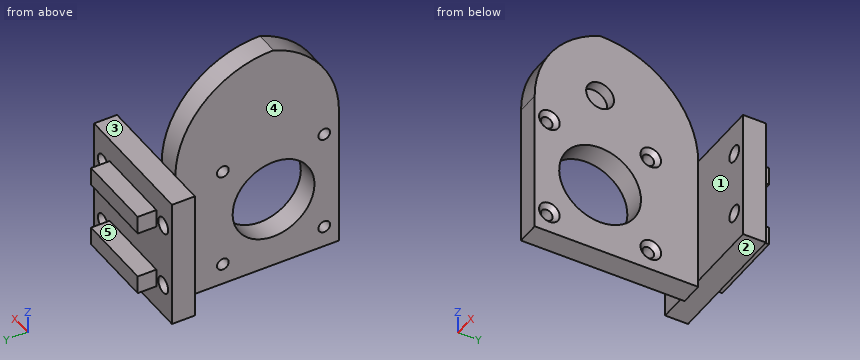
from build123d import *

# Parameters (mm, degrees)
CROQUIS1_W                                           = 40
CROQUIS1_H                                           = 40
SALIENTE_EXTRUIR1_DEPTH                              = 7
CROQUIS3_W                                           = 5.6
CROQUIS3_H                                           = 5.7
SALIENTE_EXTRUIR3_DEPTH                              = 40
CROQUIS19_W                                          = 8
CROQUIS19_H                                          = 40
CORTAR_EXTRUIR5_DEPTH                                = 5.7
CROQUIS20_R                                          = 2.5
CORTAR_EXTRUIR6_DEPTH                                = 7
CROQUIS21_W                                          = 7
CROQUIS21_H                                          = 72
SALIENTE_EXTRUIR4_DEPTH                              = 50
CROQUIS22_R                                          = 12.5
CORTAR_EXTRUIR7_DEPTH                                = 7
AVELLANADO_PARA_TORNILLO_CON_CABEZA_PLAN_D           = 3.6
AVELLANADO_PARA_TORNILLO_CON_CABEZA_PLAN_CSINK_D     = 6.3
AVELLANADO_PARA_TORNILLO_CON_CABEZA_PLAN_CSINK_ANGLE = 90
CROQUIS25_R                                          = 4.25
CORTAR_EXTRUIR8_DEPTH                                = 3.5
REDONDEO1_R                                          = 30
REDONDEO2_R                                          = 30


# Some blends are built 0.0001 mm under size
with BuildPart() as part:
    # Croquis1 → Saliente-Extruir1 (new body)
    with BuildSketch(Plane(origin=(0, 0, 0), x_dir=(1, 0, 0), z_dir=(0, 1, 0))):
        Rectangle(CROQUIS1_W, CROQUIS1_H)
    extrude(amount=SALIENTE_EXTRUIR1_DEPTH)

    # Croquis3 → Saliente-Extruir3 (add)
    with BuildSketch(Plane.ZY.offset(20)):
        with Locations((10, 9.85)):
            Rectangle(CROQUIS3_W, CROQUIS3_H)
        with Locations((-10, 9.85)):
            Rectangle(CROQUIS3_W, CROQUIS3_H)
    extrude(amount=-SALIENTE_EXTRUIR3_DEPTH)

    # Croquis19 → Cortar-Extruir5 (cut)
    with BuildSketch(Plane(origin=(0, 12.7, 0), x_dir=(1, 0, 0), z_dir=(0, 1, 0))):
        with Locations((-16, 0)):
            Rectangle(CROQUIS19_W, CROQUIS19_H)
        with Locations((16, 0)):
            Rectangle(CROQUIS19_W, CROQUIS19_H)
    extrude(amount=-CORTAR_EXTRUIR5_DEPTH, mode=Mode.SUBTRACT)

    # Croquis20 → Cortar-Extruir6 (cut)
    with BuildSketch(Plane(origin=(0, 7, 0), x_dir=(1, 0, 0), z_dir=(0, 1, 0))):
        with Locations(Location((-15.5, 10, 0), (0, 0, 270))):
            Circle(CROQUIS20_R)
        with Locations(Location((15.5, 10, 0), (0, 0, 270))):
            Circle(CROQUIS20_R)
        with Locations(Location((15.5, -10, 0), (0, 0, 270))):
            Circle(CROQUIS20_R)
        with Locations(Location((-15.5, -10, 0), (0, 0, 270))):
            Circle(CROQUIS20_R)
    extrude(amount=-CORTAR_EXTRUIR6_DEPTH, mode=Mode.SUBTRACT)

    # Croquis21 → Saliente-Extruir4 (add)
    with BuildSketch(Plane.XZ):
        with Locations((-6.5, 14)):
            Rectangle(CROQUIS21_W, CROQUIS21_H)
    extrude(amount=SALIENTE_EXTRUIR4_DEPTH)

    # Croquis22 → Cortar-Extruir7 (cut)
    with BuildSketch(Plane(origin=(-3, 0, 0), x_dir=(0, 0, -1), z_dir=(1, 0, 0))):
        with Locations((0, -30)):
            Circle(CROQUIS22_R)
    extrude(amount=-CORTAR_EXTRUIR7_DEPTH, mode=Mode.SUBTRACT)

    # Avellanado para tornillo con cabeza plana de M31 (through all)
    with Locations(Plane(origin=(-3, -14.5, 15.5), x_dir=(0, 0, 1), z_dir=(1, 0, 0))):
        with Locations((0, 0), (-31, 0), (-31, 31), (0, 31)):
            CounterSinkHole(AVELLANADO_PARA_TORNILLO_CON_CABEZA_PLAN_D / 2, AVELLANADO_PARA_TORNILLO_CON_CABEZA_PLAN_CSINK_D / 2, counter_sink_angle=AVELLANADO_PARA_TORNILLO_CON_CABEZA_PLAN_CSINK_ANGLE)

    # Croquis25 → Cortar-Extruir8 (cut)
    with BuildSketch(Plane(origin=(-3, 0, 0), x_dir=(0, 0, -1), z_dir=(1, 0, 0))):
        with Locations((-30, -30)):
            Circle(CROQUIS25_R)
    extrude(amount=-CORTAR_EXTRUIR8_DEPTH, mode=Mode.SUBTRACT)

    # Redondeo1
    redondeo1_edges = [part.edges().sort_by_distance(p)[0] for p in [
        (-6.5, 0, 50),
    ]]
    fillet(redondeo1_edges, radius=REDONDEO1_R - 0.0001)  # a hair under: the kernel refuses the full size

    # Redondeo2
    # the kernel refuses this fillet: 30 mm, written as the material it takes off along each edge
    with BuildSketch(Plane(origin=(67.710766507, -50, 50), x_dir=(0, 1, 0), z_dir=(-1, 0, 0))) as redondeo2_piece_1:
        with BuildLine():
            CenterArc((30, 28.284306603), REDONDEO2_R, 180, 70.528981937)
            Line((0, 28.284306603), (-0.6, 28.284306603))
            Line((-0.6, 28.284306603), (-0.6, 0))
            Line((-0.6, 0), (0, -0.6))
            ThreePointArc((0, -0.6), (10.00005, -0.6), (19.800102, -0.565686132))
            Line((19.800102, -0.565686132), (20.0001, 0))
        make_face()
    extrude(amount=148.421533013, mode=Mode.SUBTRACT)


solid = part.part
Here's how the part is built. I have some questions about the finished solid (model axes, mm). Face numbers are marked on the shaded views. A direction names the side the tool comes from. Coordinates: 2 decimals unless noted, no trailing zeros. Write each loop counter-clockwise with the first axis right and the second up, starting at its lowest first coordinate (ties: lowest second). Pieces come first, ordered by that corner, then holes. Notation, with made-up numbers: (-4, 49.25) - (2, 49.25) arc R17 cw to (2, 57.25) - close; hole circle Ø1 at (26, -31). An arc over 180 degrees is marked (long way). Use one line per item in the form item = value.
1) Suppose I cut it at D-D, the plane y = -14.5. Write out the boundary of the cut face in (x, z), plus the area to 3 significant figures.
Solved:
outline = (-10, -22) - (-3, -22) - (-3, -18.65) - (-4.35, -17.3) - (-10, -17.3) - close; (-10, -13.7) - (-4.35, -13.7) - (-3, -12.35) - (-3, 12.35) - (-4.35, 13.7) - (-10, 13.7) - close; (-10, 17.3) - (-4.35, 17.3) - (-3, 18.65) - (-3, 45.69) - (-10, 45.69) - close
area = 420 mm2
2) I need wall thicknesses on line 1 (X direction, y = 3, z = 10); line 2 (Y direction, x = -8, z = 0); line 3 (Z direction, x = -7.9, y = -14.5). Which ranges of each line are inside material? Lowest first, please.
Solved:
line_1 = -20 to -18, -13 to 13, 18 to 20
line_2 = -50 to -42.5, -17.5 to 7
line_3 = -22 to -17.3, -13.7 to 13.7, 17.3 to 45.69
3) On a 3-axis mill with a long thin cutter (end or side, diameter ignored), from which of +Z, -Z, +X, -X, +Y, -Y can I reach the whole of each face in a straight line? I mean the marked faces 1, 2, 3, 4 and 5. Say none if no direction works.
Solved:
face_1 = +Z, -Z, +X, -Y
face_2 = -Z, +X, -X, +Y
face_3 = +Z, +X, -X, +Y
face_4 = +Z, -Z, -X, -Y
face_5 = +X, -X, +Y
4) Suppose I cut it at C-C, the plane y = -36.5. Write out the boundary of the cut face in (x, z), plus the area to 3 significant figures.
Solved:
outline = (-10, -22) - (-3, -22) - (-3, -10.68) - (-10, -10.68) - close; (-10, 10.68) - (-3, 10.68) - (-3, 46.77) - (-10, 46.77) - close
area = 332 mm2
5) I'm going to push flat-ended pins straight in: P1, Ø6, axis at y = 8.5, z = 9, coming from the +X side; P2, Ø2, axis at y = -16, z = 40.5, coming from the +X side; P3, Ø8, axis at x = -15.5, z = -10, coming from the -Y side; P4, Ø4.5, axis at x = 5, y = 8.5, coming from the -Z side. Where does each tip first touch, or does it pass through?
Solved:
P1 = 20
P2 = -3
P3 = 0
P4 = -20
6) Suppose I cut it at A-A, the plane x = -14. Write out the boundary of the cut face in (y, z).
Solved:
outline = (0, -20) - (7, -20) - (7, -12) - (0, -12) - close; (0, -8) - (7, -8) - (7, 8) - (0, 8) - close; (0, 12) - (7, 12) - (7, 20) - (0, 20) - close
7) Suppose I cut it at B-B, the plane z = 15.5. Write out the boundary of the cut face in (x, y), plus the area to 3 significant figures.
Solved:
outline = (-20, 0) - (-10, 0) - (-10, -12.7) - (-4.35, -12.7) - (-3, -11.35) - (-3, 0) - (20, 0) - (20, 7) - (-20, 7) - close; (-10, -50) - (-3, -50) - (-3, -48.65) - (-4.35, -47.3) - (-10, -47.3) - close; (-10, -43.7) - (-4.35, -43.7) - (-3, -42.35) - (-3, -17.65) - (-4.35, -16.3) - (-10, -16.3) - close
area = 576 mm2
